Answer from the drawing. Dimensions are ordinates in mm from the lowest x, y and z of the part. A direction names the side the tool comes from. Give positions to 0.01 mm unless a question says otherwise; leave off trailing zeros. Write each loop counter-clockwise with the first axis right and the second up, starting at its lowest first coordinate (ties: lowest second). Pieces come first, ordered by that corner, then holes. Notation, with made-up numbers: M 16,59 L 59,59 A12 cw 59,70 Z; hole C -12,15 d8. An arc over 180 degrees is marked long. Answer as a JSON object with one key per item and string values.
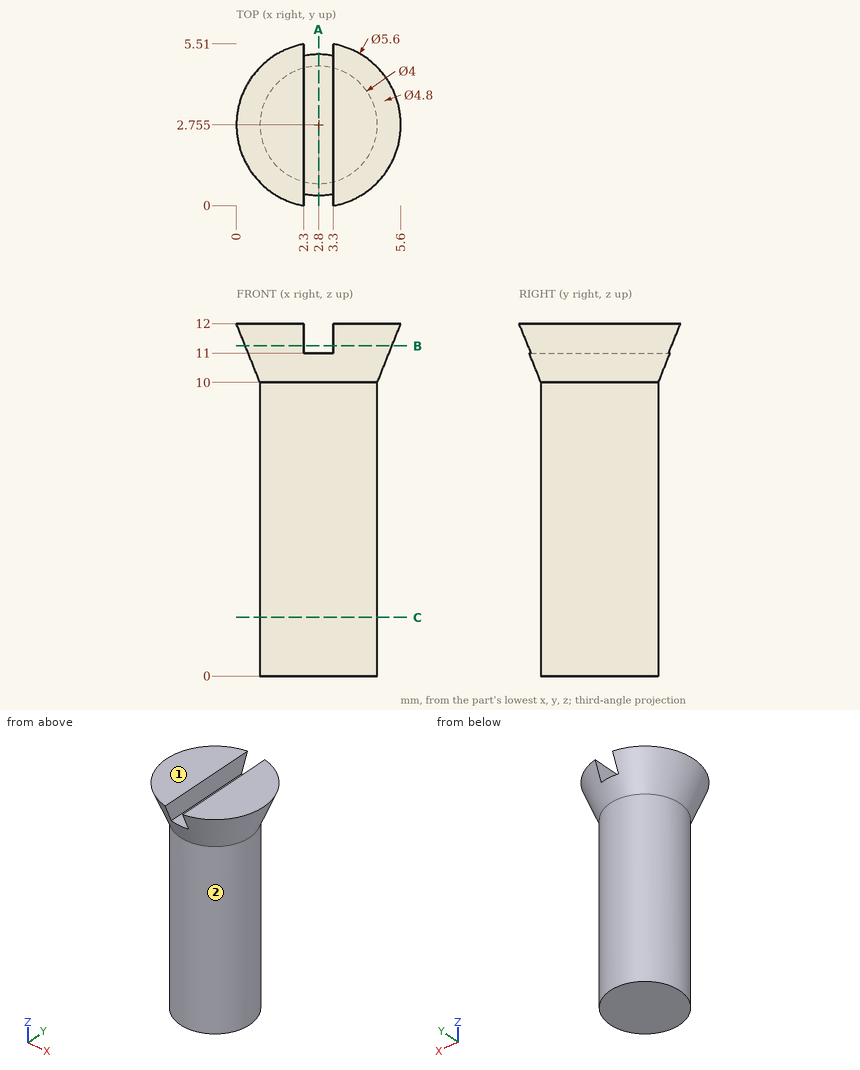
1. Consider line 1 along Z through (x, y) = (2.75, 3.3); line 2 along X through (y, z) = (2.7, 4); line 3 along X through (y, z) = (4.05, 10.5). Determine where each line is inside the solid, lowest interval first.
Verdict:
{"line 1": "z = 0 to 11", "line 2": "x = 0.8 to 4.8", "line 3": "x = 1.02 to 4.58"}
2. A cutting plane is placed at C-C, the plane z = 2. Give the vertices of the cut face in (x, y) (3 decimals).
Verdict:
{"outline": "C 2.8,2.755 d4"}
3. Flat-ended cylindrical pins translate along their axes: pin 1 (2 mm diameter, centred on y = 4, z = 3.5, fed in from +X); pin 2 (1.1 mm diameter, centred on y = 3.5, z = 11.5, fed in from +X); pin 3 (1.1 mm diameter, centred on y = 2, z = 11.5, fed in from -X). Find the tip coordinate at first contact, or state that the pin passes through.
Verdict:
{"pin 1": "stops at x = 4.78", "pin 2": "stops at x = 5.55", "pin 3": "stops at x = 0.05"}
4. A cutting plane is placed at B-B, the plane z = 11.25. Give the vertices of the cut face in (x, y) (1 decimal).
Verdict:
{"outline": "M 2.3,0.3 L 2.3,5.2 A2.5 ccw Z; M 3.3,0.3 A2.5 ccw 3.3,5.2 Z"}
5. A cutting plane is placed at A-A, the plane x = 2.8. Give the vertices of the cut face in (y, z) (3 decimals).
Verdict:
{"outline": "M 0.355,11 L 0.755,10 L 0.755,0 L 4.755,0 L 4.755,10 L 5.155,11 Z"}
6. For the marked faces 1 and 2, determine the directions among +Z, -Z, +X, -X, +Y, -Y from which every point of the face is accessible in a straight line to the end or side of a thin tool.
Verdict:
{"face 1": "+Z, +X, -X, +Y, -Y", "face 2": "-Z"}
